Can you work these out from the model? Positions are in its coordinate system, mm. A direction names the side the tool comes from. Coordinates: 2 decimals unless noted, no trailing zeros. Order: outer loops, then holes, each group sorted by start corner. A loop starts at its lowest first (then second) coordinate and runs counter-clockwise, first axis right, second up.
```python
from build123d import *

# Parameters (mm, degrees)
F0_W   = 1.5
F0_H   = 9
F0_W_2 = 3
F0_H_2 = 3


with BuildPart() as f1:
    # F0 (on Right) → F1 (revolve)
    with BuildSketch(Plane.YZ):
        Polygon((3, -4.11543), (3, -2.11543), (1.5, -2.11543), (-2, -2.11543), (-2, -4.11543), (0, -4.11543), align=None)
        with Locations((2.25, 2.38457)):
            Rectangle(F0_W, F0_H)
        with Locations((1.5, -5.61543)):
            Rectangle(F0_W_2, F0_H_2)
    revolve(axis=Axis((0, 3, 2.38457), (0, 0, 1)))


solid = f1.part
```
1. Imagine slicing it at D-D on y = 5. Please give me the cut outline in (x, z), then the cut area to 3 significant figures.
Completed:
outline: (-4.58, -4.12) - (-2.24, -4.12) - (-2.24, -7.12) - (2.24, -7.12) - (2.24, -4.12) - (4.58, -4.12) - (4.58, -2.12) - (-4.58, -2.12) - close
area: 31.7 mm2
2. On a 3-axis mill with a long thin cutter (end or side, diameter ignored), from which of +Z, -Z, +X, -X, +Y, -Y can I reach the whole of each face in a straight line? I mean faces 1 (the cylindrical face through (0, 8, -3)), 2 (the flat face through (1.2, 1.8, -2.115)), 3 (the flat face through (-3.3, 3.1, -4.115)). Say none if no direction works.
Completed:
face 1: +Z, -Z
face 2: +Z
face 3: -Z
3. Imagine slicing it at C-C on z = 3. Please give me the cut outline in (x, y), then the cut area to 3 significant figures.
Completed:
outline: circle Ø3 at (0, 3)
area: 7.07 mm2
4. Imagine slicing it at B-B on x = 0. Please give me the cut outline in (y, z).
Completed:
outline: (-2, -4.12) - (0, -4.12) - (0, -7.12) - (6, -7.12) - (6, -4.12) - (8, -4.12) - (8, -2.12) - (4.5, -2.12) - (4.5, 6.88) - (1.5, 6.88) - (1.5, -2.12) - (-2, -2.12) - close
5. I'm going to push flat-ended pins straight in: pin 1 (1 mm diameter, centred on x = 1.5, y = -0.5, fed in from -Z); pin 2 (1 mm diameter, centred on y = 1, z = -3, fed in from +X); pin 3 (4 mm diameter, centred on y = 5.5, z = 4, fed in from -X). Where does each tip first touch, or does it pass through?
Completed:
pin 1: stops at z = -4.12
pin 2: stops at x = 4.77
pin 3: stops at x = -1.41
6. Please list where these lines run through material, in increasing order: probe 1 along Z at (x, y) = (-1.75, 2.5); probe 2 along Z at (x, y) = (4.25, 3); probe 3 along Y at (x, z) = (-2, -3.5).
Completed:
probe 1: z = -7.12 to -2.12
probe 2: z = -4.12 to -2.12
probe 3: y = -1.58 to 7.58
7. Imagine slicing it at A-A on y = 3. Please give me the cut outline in (x, z).
Completed:
outline: (-5, -4.12) - (-3, -4.12) - (-3, -7.12) - (3, -7.12) - (3, -4.12) - (5, -4.12) - (5, -2.12) - (1.5, -2.12) - (1.5, 6.88) - (-1.5, 6.88) - (-1.5, -2.12) - (-5, -2.12) - close
